from build123d import *

# Parameters (mm, degrees)
SKETCH_1_W          = 35
SKETCH_1_H          = 23
EXTRUDE_1_DEPTH     = 10
SKETCH_2_W          = 23.830576701
SKETCH_2_H          = 10.361120305
CUT_EXTRUDE_1_DEPTH = 10
CUT_EXTRUDE_2_REACH = 27.1
SKETCH_3_R          = 0.875
SKETCH_4_R          = 1
EXTRUDE_2_DEPTH     = 3


with BuildPart() as part:
    # 草圖1 → 填料-伸長1 (new body)
    with BuildSketch(Plane.XY):
        with Locations((-0.640978345, -2.673693694)):
            Rectangle(SKETCH_1_W, SKETCH_1_H)
    extrude(amount=EXTRUDE_1_DEPTH)

    # 草圖2 → 除料-伸長1 (cut)
    with BuildSketch(Plane.XY.offset(10)):
        with Locations((-0.14284756, -2.713544157)):
            Rectangle(SKETCH_2_W, SKETCH_2_H)
    extrude(amount=-CUT_EXTRUDE_1_DEPTH, mode=Mode.SUBTRACT)

    # 草圖3 → 除料-伸長2 (cut, up to next)
    with BuildSketch(Plane.XY.offset(10), mode=Mode.PRIVATE) as cut_extrude_2_sk1:
        with Locations((-16.665978345, 3.551306306)):
            Circle(SKETCH_3_R)
    cut_extrude_2_tool1 = extrude(cut_extrude_2_sk1.sketch, amount=-CUT_EXTRUDE_2_REACH, mode=Mode.PRIVATE) & part.part
    # 草圖3 → 除料-伸長2 (cut, up to next)
    with BuildSketch(Plane.XY.offset(10), mode=Mode.PRIVATE) as cut_extrude_2_sk2:
        with Locations((15.284021655, -12.638693694)):
            Circle(SKETCH_3_R)
    cut_extrude_2_tool2 = extrude(cut_extrude_2_sk2.sketch, amount=-CUT_EXTRUDE_2_REACH, mode=Mode.PRIVATE) & part.part
    add(cut_extrude_2_tool1.solids().sort_by_distance((-16.665978, 3.551306, 10))[0], mode=Mode.SUBTRACT)
    add(cut_extrude_2_tool2.solids().sort_by_distance((15.284022, -12.638694, 10))[0], mode=Mode.SUBTRACT)

    # 草圖4 → 填料-伸長2 (add)
    with BuildSketch(Plane.XY.offset(10)):
        with Locations((-15.547323348, 6.81929444)):
            Circle(SKETCH_4_R)
        with Locations((-13.047323348, 6.81929444)):
            Circle(SKETCH_4_R)
        with Locations((-10.547323348, 6.81929444)):
            Circle(SKETCH_4_R)
        with Locations((-8.047323348, 6.81929444)):
            Circle(SKETCH_4_R)
    extrude(amount=EXTRUDE_2_DEPTH)


solid = part.part
Design review of the part built by this model. Coordinates are the model's own, in mm. A direction names the side the tool comes from. Coordinates: 2 decimals unless noted, no trailing zeros. Loops run counter-clockwise (first coordinate to the right, second up) from the corner with the lowest first, then second, coordinate; pieces in that order, holes last. Notation, with made-up numbers: M -10,-12 L 3,-12 A26 ccw 3,15 Z; hole C 63.25,-40 d10. An arc over 180 degrees is marked long. Use one line per item in the form item = value.
(1) For line 1 along Y through (x, z) = (1.5, 7); line 2 along X through (y, z) = (1.75, 6.5); line 3 along X through (y, z) = (3.5, 1.25), list the stretches that pass through material, from the lowest coordinate up. Write a range as from..to.
Return value:
line_1 = -14.17..-7.89, 2.47..8.83
line_2 = -18.14..-12.06, 11.77..16.86
line_3 = -18.14..-17.54, -15.79..16.86
(2) Draft analysis for pull direction Y (two halves, no side actions). For faces 4 (the face through (-1, 3, 10)), 5 (the face through (-10.01, 7.662, 11.479)), 6 (the face through (11.772, -3, 5)), state which applies: pulls with the +Y half, pulls with the -Y half, needs draft (parallel to the pull), parting line crosses it, or undercut.
Return value:
face_4 = needs draft
face_5 = parting line crosses it
face_6 = undercut
(3) Consider section C-C (z = 8.5). Write out the cut boundary in (x, y) (3 decimals), and give its area (3 significant figures).
Return value:
outline = M -18.141,-14.174 L 16.859,-14.174 L 16.859,8.826 L -18.141,8.826 Z; hole C -16.666,3.551 d1.75; hole M -12.058,-7.894 L 11.772,-7.894 L 11.772,2.467 L -12.058,2.467 Z; hole C 15.284,-12.639 d1.75
area = 553 mm2
(4) Consider section B-B (y = -7.5). Write out the cut boundary in (x, z), and give its area (3 significant figures).
Return value:
outline = M -18.14,0 L -12.06,0 L -12.06,10 L -18.14,10 Z; M 11.77,0 L 16.86,0 L 16.86,10 L 11.77,10 Z
area = 112 mm2
(5) Consider section D-D (x = -13). Write out the cut boundary in (y, z).
Return value:
outline = M -14.17,0 L 8.83,0 L 8.83,10 L 7.82,10 L 7.82,13 L 5.82,13 L 5.82,10 L -14.17,10 Z
(6) For faces 1 (the face through (-12.058, -3, 5)), 2 (the face through (-16, 7, 13)), 3 (the face through (-7.094, 7.12, 11.479)), list the 3-axis set-ups (+Z, -Z, +X, -X, +Y, -Y) from which the entire face can be reached by the end or side of a thin tool; tool diameter is ignored.
Return value:
face_1 = +Z, -Z
face_2 = +Z, +X, -X, +Y, -Y
face_3 = +Z
(7) Clearance check with flat-ended pins moving along their axes: P1, Ø2, axis at x = -10.5, z = 11.5, coming from the -Y side; P2, Ø7, axis at x = -8, y = -5, coming from the +Z side. State where each tip first meets the part, or that it passes through.
Return value:
P1 = 5.82
P2 = 10
(8) Consider section A-A (x = 0). Write out the cut boundary in (y, z), and give its area (3 significant figures).
Return value:
outline = M -14.17,0 L -7.89,0 L -7.89,10 L -14.17,10 Z; M 2.47,0 L 8.83,0 L 8.83,10 L 2.47,10 Z
area = 126 mm2
